Geometry: final body of the model. Coordinates: model frame, mm. Face numbers are marked on the shaded views. A direction names the side the tool comes from. Give positions to 0.01 mm unless a question says otherwise; leave off trailing zeros. Loops run counter-clockwise (first coordinate to the right, second up) from the corner with the lowest first, then second, coordinate; pieces in that order, holes last.
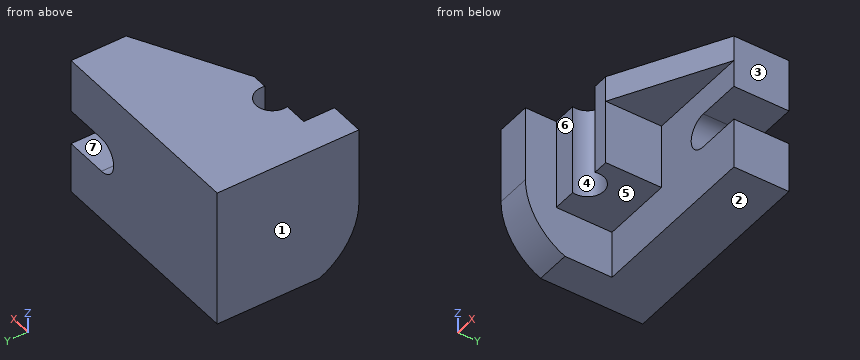
from build123d import *

# Parameters (mm, degrees)
F0_W     = 96
F0_H     = 64
F1_DEPTH = 25.4
F2_W     = 20
F2_H     = 16
F3_DEPTH = 25.4
F5_DEPTH = 16
F7_DEPTH = 42
F9_DEPTH = 12


with BuildPart() as f1:
    # F0 (on Front) → F1 (new body)
    with BuildSketch(Plane.XZ):
        with Locations((-0.479123, -7.401277)):
            Rectangle(F0_W, F0_H)
    extrude(amount=F1_DEPTH)

    # F2 (on face) → F3 (cut)
    with BuildSketch(Plane.XZ.offset(25.4)):
        with BuildLine():
            Line((27.520877, -16), (27.520877, 0))
            ThreePointArc((27.520877, 0), (19.520877, -8), (27.520877, -16))
        make_face()
        with Locations((37.520877, -8)):
            Rectangle(F2_W, F2_H)
    extrude(amount=-F3_DEPTH, mode=Mode.SUBTRACT)

    # F4 (on face) → F5 (join)
    with BuildSketch(Plane(origin=(-48.479123, 0, 0), x_dir=(0, -1, 0), z_dir=(-1, 0, 0))):
        with BuildLine():
            Line((65.310675, 24.598723), (25.4, 24.598723))
            Line((25.4, 24.598723), (25.4, -39.401277))
            Line((25.4, -39.401277), (47.101744, -39.401277))
            ThreePointArc((47.101744, -39.401277), (60.378314, -27.594341), (65.310675, -10.525571))
            Line((65.310675, -10.525571), (65.310675, 24.598723))
        make_face()
    extrude(amount=-F5_DEPTH)

    # F6 (on face) → F7 (join)
    with BuildSketch(Plane.XY.offset(24.598723)):
        with BuildLine():
            Line((0, -25.4), (-32.479123, -25.4))
            Line((-32.479123, -25.4), (-32.479123, -51.092945))
            Line((-32.479123, -51.092945), (-21.691002, -51.092945))
            ThreePointArc((-21.691002, -51.092945), (-14.349926, -41.873779), (-7.008849, -51.092945))
            Line((-7.008849, -51.092945), (0, -51.092945))
            Line((0, -51.092945), (0, -25.4))
        make_face()
    extrude(amount=-F7_DEPTH)

    # F8 (on face) → F9 (join)
    with BuildSketch(Plane.XY.offset(24.598723)):
        Polygon((0, -51.092945), (47.520877, -25.4), (0, -25.4), align=None)
    extrude(amount=-F9_DEPTH)


solid = f1.part
Item 1: Section query D-D on y = -22. Return loops of the section in (x, z), plus the area to 3 significant figures.
Values follow:
outline: (-48.48, -39.4) - (47.52, -39.4) - (47.52, -16) - (27.52, -16) arc R8 cw to (27.52, 0) - (47.52, 0) - (47.52, 24.6) - (-48.48, 24.6) - close
area: 5,720 mm2
Item 2: Draft query along X for the marked faces 1, 2, 3 and 4. Return one class per face: +X half, -X half, draft (parallel to the pull), parting line (faces both ways), or undercut.
Values follow:
face 1: -X half
face 2: draft
face 3: +X half
face 4: undercut
Item 3: Set-up query: the marked faces 5, 6 and 7. Return all of +Z, -Z, +X, -X, +Y, -Y with unobstructed straight access to the full face (end or side cutting, diameter ignored); none if empty.
Values follow:
face 5: -Z, +X, -Y
face 6: +Z, -Z, +X, -Y
face 7: +X, +Y, -Y
Item 4: Section query A-A on y = -49.5. Return loops of the section in (x, z), plus the area to 3 significant figures.
Values follow:
outline: (-48.48, -38.13) - (-32.48, -38.13) - (-32.48, -17.4) - (-21.88, -17.4) - (-21.88, 24.6) - (-48.48, 24.6) - close; (-6.82, -17.4) - (0, -17.4) - (0, 12.6) - (2.95, 12.6) - (2.95, 24.6) - (-6.82, 24.6) - close
area: 1,770 mm2
Item 5: Ray query, probe 1 along X at (y, z) = (-49, -10); probe 2 along Z at (x, y) = (29, -24.5); probe 3 along Y at (x, z) = (31.5, -31.5). Return the intervals inside material, ascending.
Values follow:
probe 1: x = -48.48 to -21.87, -6.83 to 0
probe 2: z = -39.4 to -16, 0 to 24.6
probe 3: y = -25.4 to 0
Item 6: Section query B-B on x = 29. Return loops of the section in (y, z), plus the area to 3 significant figures.
Values follow:
outline: (-35.41, 12.6) - (-25.4, 12.6) - (-25.4, 0) - (0, 0) - (0, 24.6) - (-35.41, 24.6) - close; (-25.4, -39.4) - (0, -39.4) - (0, -16) - (-25.4, -16) - close
area: 1,340 mm2
Item 7: Pin query (flat end, axial travel): pin 1 (7.5 mm diameter, centred on x = -12, y = -43, fed in from -Z); pin 2 (4 mm diameter, centred on x = -24.5, z = -32.5, fed in from -Y); pin 3 (10 mm diameter, centred on y = -56.5, z = -4.5, fed in from +X). Return the tip coordinate at first contact, or that it passes through.
Values follow:
pin 1: stops at z = -17.4
pin 2: stops at y = -25.4
pin 3: stops at x = -32.48
Item 8: Section query C-C on x = -28.5. Return loops of the section in (y, z), plus the area to 3 significant figures.
Values follow:
outline: (-51.09, -17.4) - (-25.4, -17.4) - (-25.4, -39.4) - (0, -39.4) - (0, 24.6) - (-51.09, 24.6) - close
area: 2,700 mm2
